Autodesk Inventor part; units mm, degrees
ref_plane "YZ Plane" through (0, 0, 0) normal (1, 0, 0) x (0, 1, 0)
ref_plane "XZ Plane" through (0, 0, 0) normal (0, 1, 0) x (-1, 0, 0)
ref_plane "XY Plane" through (0, 0, 0) normal (0, 0, 1) x (1, 0, 0)
sketch "Sketch1" plane through (0, 0, 0) normal (0, 0, 1) x (1, 0, 0)
  line L0 (-21.1, -21.1) -> (21.1, -21.1)
  line L1 (21.1, -21.1) -> (21.1, 21.1)
  line L2 (21.1, 21.1) -> (-21.1, 21.1)
  line L3 (-21.1, 21.1) -> (-21.1, -21.1)
  line L4 (-21.1, -21.1) -> (21.1, 21.1) construction
  line L5 (21.1, -21.1) -> (-21.1, 21.1) construction
  line L6 (-23.5, 23.5) -> (23.5, 23.5)
  line L7 (23.5, 23.5) -> (23.5, -23.5)
  line L8 (23.5, -23.5) -> (-23.5, -23.5)
  line L9 (-23.5, -23.5) -> (-23.5, 23.5)
  line L10 (-23.5, 23.5) -> (23.5, -23.5) construction
  line L11 (23.5, 23.5) -> (-23.5, -23.5) construction
  line L12 (-5, -21.1) -> (-5, -23.5)
  line L13 (5, -21.1) -> (5, -23.5)
  circle A0 centre (8, 8) radius 1.8
  circle A1 centre (8, -8) radius 1.8
  circle A2 centre (-8, -8) radius 1.8
  circle A3 centre (-8, 8) radius 1.8
  line L14 (-11, 11) -> (11, -11) construction
  line L15 (11, 11) -> (-11, -11) construction
  circle A4 centre (0, 0) radius 4
  circle A5 centre (-8, 8) radius 2.75
  circle A6 centre (-8, -8) radius 2.75
  circle A7 centre (8, 8) radius 2.75
  circle A8 centre (8, -8) radius 2.75
  dimension "d0" = 42.2
  dimension "d1" = 42.2
  dimension "d2" = 47
  dimension "d3" = 47
  dimension "d4" = 10
  dimension "d5" = 5
  dimension "d6" = 3.6
  dimension "d7" = 3.6
  dimension "d8" = 3.6
  dimension "d9" = 3.6
  dimension "d10" = 16
  dimension "d11" = 16
  dimension "d12" = 16
  dimension "d13" = 8
  dimension "d20" = 8
  dimension "d21" = 5.5
  dimension "d22" = 5.5
  dimension "d23" = 5.5
  dimension "d24" = 5.5
extrude "Extrusion1" add sketch "Sketch1" along normal blind 8.5 contours L0 L12 L8 L9 L6 L7 L13 L1 L2 L3
extrude "Extrusion2" add sketch "Sketch1" along normal blind 1.5 contours L3 L2 L1 L0 | L0 L13 L8 L12 | A0 | A1 | A2 | A3 | A5 | A6 | A7 | A8
extrude "Extrusion3" add sketch "Sketch1" against normal blind 4 contours A0 | A1 | A2 | A3 | A5 | A6 | A7 | A8
extrude "Extrusion4" add sketch "Sketch1" against normal blind 6 contours A0 | A1 | A2 | A3
properties part number "MagEncHolder"
Work out the finished part from the listing and answer in its coordinate system (mm). A direction names the side the tool comes from. Round coordinates to 2 decimals unless told otherwise and drop trailing zeros. Order: outer loops, then holes, each group sorted by start corner. A loop starts at its lowest first (then second) coordinate and runs counter-clockwise, first axis right, second up. Notation, with made-up numbers: M 55.5,80 L 91.5,80 A18 ccw 91.5,107 Z; hole C 70.5,15.25 d7. An arc over 180 degrees is marked long. Put each result on its own line as item: value. Start each with the question number.
Q1. Straight lines are drawn through the part: L1, parallel to X at y = 16, z = 2.75; L2, parallel to Z at x = -6.5, y = 7.5. For each, find the intervals that lie inside material, in ascending order. Write a range as [from, to].
Q2. Section B-B, the plane y = 0 is taken. Write down the section's boundary in (x, z), and give its area (3 significant figures).
Q3. Flat-ended cylindrical pins translate along their axes: pin 1 (21 mm diameter, centred on x = 3.5, y = 1.5, fed in from +Z); pin 2 (4 mm diameter, centred on y = -8.5, z = -3, fed in from +X); pin 3 (3.5 mm diameter, centred on x = -2, z = 6.5, fed in from -Y); pin 4 (23.5 mm diameter, centred on x = -4.5, y = 2.5, fed in from -Z). Find the tip coordinate at first contact, or state that the pin passes through.
Q4. Section C-C, the plane z = 4.25 is taken. Write down the section's boundary in (x, y).
Q5. For a pull along X with two mould halves and no side action, classify faces 6 (the flat face through (0, 23, 8.5)), 7 (the cylindrical face through (-5.46, 6.95, -1.97)), 8 (the flat face through (-23.5, 0, 4)) as pulls with the +X half, pulls with the -X half, needs draft (parallel to the pull), parting line crosses it, or undercut.
Q6. A tool of negligible diameter and unlimited length cuts with its end or side. For faces 1 (the flat face through (21.1, 0, 5)), 2 (the cylindrical face through (7.61, -9.757, -4.986)), 3 (the flat face through (0, 23.5, 4)), 4 (the flat face through (23.5, 0, 4)), 5 (the flat face through (5, -22, 5)), from which of +Z, -Z, +X, -X, +Y, -Y can it reach the whole face along a straight path? Write none if from no direction.
Q7. Section A-A, the plane x = 0 is taken. Write down the section's boundary in (y, z), and give its area (3 significant figures).
Q8. Section D-D, the plane x = -8 is taken. Write down the section's boundary in (y, z), and give its area (4 significant figures).
Findings below:
1. L1: x = [-23.5, -21.1], [21.1, 23.5]
1. L2: z = [-6, 1.5]
2. outline: M -23.5,0 L -4,0 L -4,1.5 L -21.1,1.5 L -21.1,8.5 L -23.5,8.5 Z; M 4,0 L 23.5,0 L 23.5,8.5 L 21.1,8.5 L 21.1,1.5 L 4,1.5 Z
2. area: 92.1 mm^2
3. pin 1: stops at z = 1.5
3. pin 2: stops at x = 10.75
3. pin 3: stops at y = 21.1
3. pin 4: stops at z = -6
4. outline: M -23.5,-23.5 L -5,-23.5 L -5,-21.1 L -21.1,-21.1 L -21.1,21.1 L 21.1,21.1 L 21.1,-21.1 L 5,-21.1 L 5,-23.5 L 23.5,-23.5 L 23.5,23.5 L -23.5,23.5 Z
5. face 6: needs draft
5. face 7: undercut
5. face 8: pulls with the -X half
6. face 1: +Z
6. face 2: -Z
6. face 3: +Z, -Z, +X, -X, +Y
6. face 4: +Z, -Z, +X, +Y, -Y
6. face 5: +Z, -Y
7. outline: M -23.5,0 L -4,0 L -4,1.5 L -23.5,1.5 Z; M 4,0 L 23.5,0 L 23.5,8.5 L 21.1,8.5 L 21.1,1.5 L 4,1.5 Z
7. area: 75.3 mm^2
8. outline: M -23.5,0 L -10.75,0 L -10.75,-4 L -9.8,-4 L -9.8,-6 L -6.2,-6 L -6.2,-4 L -5.25,-4 L -5.25,0 L 5.25,0 L 5.25,-4 L 6.2,-4 L 6.2,-6 L 9.8,-6 L 9.8,-4 L 10.75,-4 L 10.75,0 L 23.5,0 L 23.5,8.5 L 21.1,8.5 L 21.1,1.5 L -21.1,1.5 L -21.1,8.5 L -23.5,8.5 Z
8. area: 162.5 mm^2
